Could you check a few things on this model? Use its own coordinates, in mm. Face numbers are marked on the shaded views. Give positions to 0.01 mm unless a question says otherwise; leave off trailing zeros. Order: outer loops, then holes, each group sorted by start corner. A loop starts at its lowest first (then second) coordinate and runs counter-clockwise, first axis right, second up. Notation, with made-up numbers: (12.25, 21.5) - (66.25, 21.5) arc R20 cw to (66.25, 40.5) - close; hole circle Ø2 at (58.25, -22). An arc over 180 degrees is marked (long way). Put each result on its own line as item: value.
from build123d import *

# Parameters (mm, degrees)
SKETCH1_R           = 17.9
BOSS_EXTRUDE1_DEPTH = 54.51
SKETCH2_R           = 12.5735
BOSS_EXTRUDE2_DEPTH = 3.3
SKETCH4_R           = 11
CUT_EXTRUDE2_DEPTH  = 59.3


with BuildPart() as part:
    # Sketch1 → Boss-Extrude1 (new body)
    with BuildSketch(Plane(origin=(0, 0, 0), x_dir=(1, 0, 0), z_dir=(0, 1, 0))):
        Circle(SKETCH1_R)
    extrude(amount=BOSS_EXTRUDE1_DEPTH)

    # Sketch2 → Boss-Extrude2 (add)
    with BuildSketch(Plane(origin=(0, 54.51, 0), x_dir=(1, 0, 0), z_dir=(0, 1, 0))):
        Circle(SKETCH2_R)
    extrude(amount=BOSS_EXTRUDE2_DEPTH)

    # Sketch4 → Cut-Extrude2 (cut)
    with BuildSketch(Plane.XZ):
        Circle(SKETCH4_R)
    extrude(amount=-CUT_EXTRUDE2_DEPTH, mode=Mode.SUBTRACT)


solid = part.part
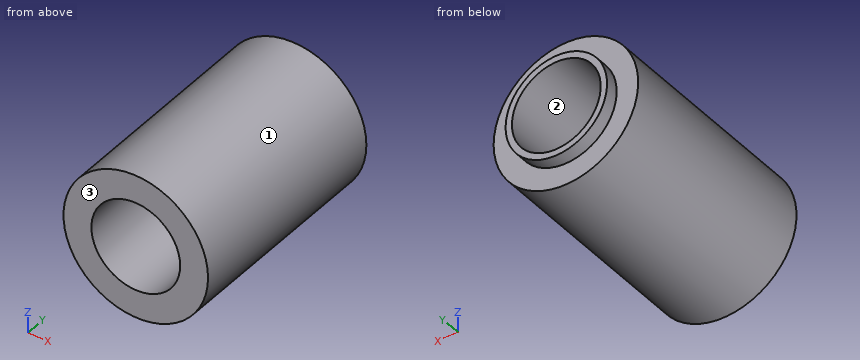
1) If I drill on line 1 (Z direction, x = 0, y = 35.5); line 2 (Y direction, x = -14.5, z = -10); line 3 (Z direction, x = 10, y = 45), over which ranges is the centre line in solid material (lowest first)? Write a range as [from, to].
Filled in:
line 1: z = [-17.9, -11], [11, 17.9]
line 2: y = [0, 54.51]
line 3: z = [-14.85, -4.58], [4.58, 14.85]
2) Suppose I cut it at A-A, the plane x = 0. List the corners of the cut face in (y, z) for me.
Filled in:
outline: (0, -17.9) - (54.51, -17.9) - (54.51, -12.57) - (57.81, -12.57) - (57.81, -11) - (0, -11) - close; (0, 11) - (57.81, 11) - (57.81, 12.57) - (54.51, 12.57) - (54.51, 17.9) - (0, 17.9) - close
3) I'm going to push flat-ended pins straight in: pin 1 (8 mm diameter, centred on x = -3, y = 41.5, fed in from +Z); pin 2 (17.5 mm diameter, centred on x = 0, z = 0, fed in from -Y); pin 3 (4 mm diameter, centred on x = -8, y = 12.5, fed in from +Z); pin 4 (6 mm diameter, centred on y = 47.5, z = -10.5, fed in from -X). Where does each tip first touch, or does it pass through?
Filled in:
pin 1: stops at z = 17.9
pin 2: passes through
pin 3: stops at z = 16.86
pin 4: stops at x = -16.25
4) We'd pull the mould along X, two halves only. Please class the marked faces 1, 2 and 3: pulls with the +X half, pulls with the -X half, needs draft (parallel to the pull), parting line crosses it, or undercut.
Filled in:
face 1: parting line crosses it
face 2: undercut
face 3: needs draft
5) Suppose I cut it at B-B, the plane z = 0. List the corners of the cut face in (x, y) for me, and give its area (3 significant figures).
Filled in:
outline: (-17.9, 0) - (-11, 0) - (-11, 57.81) - (-12.57, 57.81) - (-12.57, 54.51) - (-17.9, 54.51) - close; (11, 0) - (17.9, 0) - (17.9, 54.51) - (12.57, 54.51) - (12.57, 57.81) - (11, 57.81) - close
area: 763 mm^2
6) Suppose I cut it at D-D, the plane z = 14.5. List the corners of the cut face in (x, y) for me.
Filled in:
outline: (-10.5, 0) - (10.5, 0) - (10.5, 54.51) - (-10.5, 54.51) - close
7) Suppose I cut it at C-C, the plane y = 6.5. List the corners of the cut face in (x, z) for me.
Filled in:
outline: circle Ø35.8 at (0, 0); hole circle Ø22 at (0, 0)
